Geometry: final body of the model. Coordinates: model frame, mm. Face numbers are marked on the shaded views. A direction names the side the tool comes from. Give positions to 0.01 mm unless a question says otherwise; leave off trailing zeros. Loops run counter-clockwise (first coordinate to the right, second up) from the corner with the lowest first, then second, coordinate; pieces in that order, holes last. Notation, with made-up numbers: (-21.5, 76) - (4.5, 76) arc R31 ccw to (4.5, 107) - close; hole circle Ø11 at (76.25, 40.5). An arc over 180 degrees is marked (long way). Use CSV: the item, a comma, the result in double quotes. Start each with the question number.
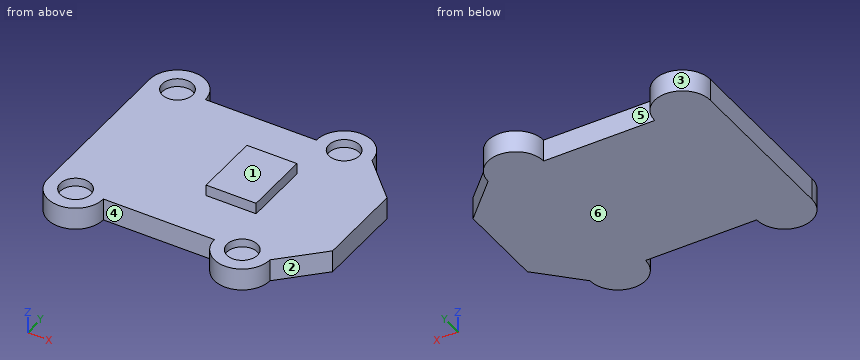
Autodesk Fusion 360 part; units mm, degrees
sketch "Colour Sensor Cover" plane through (0, 0, 0) normal (0, 0, 1) x (1, 0, 0)
  line L0 (0, 0) -> (47, 0)
  line L1 (47, 0) -> (47, 30)
  line L2 (47, 30) -> (0, 30)
  line L3 (0, 30) -> (0, 0)
  circle A0 centre (5, 30) radius 5
  circle A1 centre (35, 30) radius 5
  circle A2 centre (5, 0) radius 5
  circle A3 centre (35, 0) radius 5
  dimension "d1" = 47
  dimension "d2" = 30
  dimension "d3" = 10
  dimension "d4" = 10
  dimension "d5" = 10
  dimension "d6" = 10
  dimension "d7" = 5
  dimension "d8" = 5
  dimension "d9" = 12
  dimension "d10" = 12
extrude "Extrude1" add sketch "Colour Sensor Cover" along normal blind 4
chamfer "Chamfer1" distance 7 angle 45 2 edges at (47, 0, 2) (47, 30, 2)
sketch "Magnet Holes" plane through (0, 0, 4) normal (0, 0, 1) x (-1, 0, 0)
  line L0 (-47, -23) -> (-40, -30)
  arc A0 (-40, -30) -> (-30, -30) centre (-35, -30) ccw
  line L1 (-30, -30) -> (-10, -30)
  arc A1 (-10, -30) -> (0, -30) centre (-5, -30) ccw
  line L2 (0, -30) -> (0, 0)
  arc A2 (0, 0) -> (-10, 0) centre (-5, 0) ccw
  line L3 (-10, 0) -> (-30, 0)
  arc A3 (-30, 0) -> (-40, 0) centre (-35, 0) ccw
  line L4 (-40, 0) -> (-47, -7)
  line L5 (-47, -7) -> (-47, -23)
  circle A4 centre (-5, -30) radius 2.75
  circle A5 centre (-35, -30) radius 2.75
  circle A6 centre (-5, 0) radius 2.75
  circle A7 centre (-35, 0) radius 2.75
  dimension "d14" = 5.5
  dimension "d15" = 5.5
  dimension "d16" = 5.5
  dimension "d17" = 5.5
extrude "Extrude2" cut sketch "Magnet Holes" against normal blind 1.5 contours A4 | A5 | A6 | A7
sketch "Colour Sensor Support" plane through (0, 0, 4) normal (0, 0, 1) x (-1, 0, 0)
  circle A0 centre (-5, -30) radius 2.75
  circle A1 centre (-35, -30) radius 2.75
  circle A2 centre (-5, 0) radius 2.75
  circle A3 centre (-35, 0) radius 2.75
  line L0 (-47, -23) -> (-40, -30)
  arc A4 (-40, -30) -> (-30, -30) centre (-35, -30) ccw
  line L1 (-30, -30) -> (-10, -30)
  arc A5 (-10, -30) -> (0, -30) centre (-5, -30) ccw
  line L2 (0, -30) -> (0, 0)
  arc A6 (0, 0) -> (-10, 0) centre (-5, 0) ccw
  line L3 (-10, 0) -> (-30, 0)
  arc A7 (-30, 0) -> (-40, 0) centre (-35, 0) ccw
  line L4 (-40, 0) -> (-47, -7)
  line L5 (-47, -7) -> (-47, -23)
  line L6 (-23, -21) -> (-32, -21)
  line L7 (-32, -21) -> (-32, -9)
  line L8 (-32, -9) -> (-23, -9)
  line L9 (-23, -9) -> (-23, -21)
  dimension "d20" = 9
  dimension "d21" = 9
  dimension "d22" = 15
  dimension "d23" = 9
  dimension "d24" = 12
extrude "Extrude3" add sketch "Colour Sensor Support" along normal blind 2 contours L6 L7 L8 L9
equation "d9 = 7 mm + 5 mm"
equation "d10 = 7 mm + 5 mm"
Item 1: Pin query (flat end, axial travel): pin 1 Ø3 at (x, z) = (32, 5) entering from +Y; pin 2 Ø6 at (x, y) = (6.5, 30.5) entering from +Z; pin 3 Ø3 at (x, z) = (39.5, 0.5) entering from +Y. Return the tip coordinate at first contact, or that it passes through.
Item 2: Section D-D (y = 18). Output: boundary loops of the cut face in (x, z), plus the area to 3 significant figures.
Item 3: Section B-B (y = 32). Output: boundary loops of the cut face in (x, z).
Item 4: Ray query, probe 1 along Y at (x, z) = (5, 3.1); probe 2 along Z at (x, y) = (42, 21); probe 3 along Y at (x, z) = (25, 5.65). Return the intervals inside material, ascending.
Item 5: Reachability of the marked faces 4, 5 and 6 from +Z, -Z, +X, -X, +Y, -Y: full face, straight path, thin tool, end or side. Return the list, or none.
Item 6: Section A-A (x = 35). Output: boundary loops of the cut face in (y, z).
Item 7: Mould query, pull axis X, two halves, no side actions, for the marked faces 1, 2 and 3. Classes: pulls with the +X half, pulls with the -X half, needs draft (parallel to the pull), parting line crosses it, or undercut.
Outcome:
1,pin 1,"stops at y = 34.63"
1,pin 2,"stops at z = 4"
1,pin 3,"stops at y = 34"
2,outline,"(0, 0) - (47, 0) - (47, 4) - (32, 4) - (32, 6) - (23, 6) - (23, 4) - (0, 4) - close"
2,area,"206 mm2"
3,outline,"(0.42, 0) - (9.58, 0) - (9.58, 4) - (6.89, 4) - (6.89, 2.5) - (3.11, 2.5) - (3.11, 4) - (0.42, 4) - close; (30.42, 0) - (39.58, 0) - (39.58, 4) - (36.89, 4) - (36.89, 2.5) - (33.11, 2.5) - (33.11, 4) - (30.42, 4) - close"
4,probe 1,"y = -5 to -2.75, 2.75 to 27.25, 32.75 to 35"
4,probe 2,"z = 0 to 4"
4,probe 3,"y = 9 to 21"
5,face 4,"+Z, -Z, -Y"
5,face 5,"+Z, -Z, +Y"
5,face 6,"-Z, +X, -X, +Y, -Y"
6,outline,"(-5, 0) - (35, 0) - (35, 4) - (32.75, 4) - (32.75, 2.5) - (27.25, 2.5) - (27.25, 4) - (2.75, 4) - (2.75, 2.5) - (-2.75, 2.5) - (-2.75, 4) - (-5, 4) - close"
7,face 1,"needs draft"
7,face 2,"pulls with the +X half"
7,face 3,"undercut"
